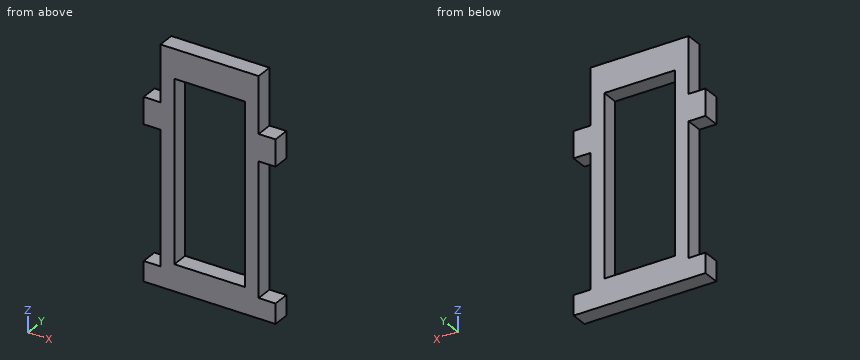
```python
from build123d import *

# Parameters (mm, degrees)
SKETCH1_W           = 53.15
SKETCH1_H           = 135.7
BOSS_EXTRUDE1_DEPTH = 6.35


with BuildPart() as part:
    # Sketch1 → Boss-Extrude1 (new, symmetric)
    with BuildSketch(Plane(origin=(0, 0, 0), x_dir=(1, 0, 0), z_dir=(0, 1, 0))):
        Polygon((-37, -88.675), (-37, -46.325), (-49.7, -46.325), (-49.7, -26.325), (-37, -26.325), (-37, 73.675), (-49.7, 73.675), (-49.7, 88.675), (49.7, 88.675), (49.7, 73.675), (37, 73.675), (37, -26.325), (49.7, -26.325), (49.7, -46.325), (37, -46.325), (37, -88.675), align=None)
        with Locations((0, 1)):
            Rectangle(SKETCH1_W, SKETCH1_H, mode=Mode.SUBTRACT)
    extrude(amount=BOSS_EXTRUDE1_DEPTH, both=True)


solid = part.part
```
Could you check a few things on this model? Use its own coordinates, in mm. Give positions to 0.01 mm unless a question says otherwise; leave off trailing zeros. Loops run counter-clockwise (first coordinate to the right, second up) from the corner with the lowest first, then second, coordinate; pieces in that order, holes last. Notation, with made-up numbers: (7.5, -30) - (28.5, -30) arc R26 cw to (28.5, 1) - close; hole circle Ø9 at (-4.75, 2). An arc over 180 degrees is marked (long way). Use one line per item in the form item = value.
1. I want a section at A-A (y = 2.5). Please give me the cut outline in (x, z) (3 decimals), and give its area (3 significant figures).
Response values:
outline = (-49.7, -88.675) - (49.7, -88.675) - (49.7, -73.675) - (37, -73.675) - (37, 26.325) - (49.7, 26.325) - (49.7, 46.325) - (37, 46.325) - (37, 88.675) - (-37, 88.675) - (-37, 46.325) - (-49.7, 46.325) - (-49.7, 26.325) - (-37, 26.325) - (-37, -73.675) - (-49.7, -73.675) - close; hole (-26.575, -68.85) - (26.575, -68.85) - (26.575, 66.85) - (-26.575, 66.85) - close
area = 6,800 mm²
2. I want a section at C-C (z = 28.5). Please give me the cut outline in (x, y) (3 decimals), and give its area (3 significant figures).
Response values:
outline = (-49.7, -6.35) - (-26.575, -6.35) - (-26.575, 6.35) - (-49.7, 6.35) - close; (26.575, -6.35) - (49.7, -6.35) - (49.7, 6.35) - (26.575, 6.35) - close
area = 587 mm²
3. I want a section at B-B (x = -41). Please give me the cut outline in (y, z) (3 decimals).
Response values:
outline = (-6.35, -88.675) - (6.35, -88.675) - (6.35, -73.675) - (-6.35, -73.675) - close; (-6.35, 26.325) - (6.35, 26.325) - (6.35, 46.325) - (-6.35, 46.325) - close
4. I'm going to push flat-ended pins straight in: pin 1 Ø4 at (y, z) = (1.5, -42.5) entering from +X; pin 2 Ø4 at (y, z) = (-1.5, -26.5) entering from -X; pin 3 Ø4 at (x, y) = (-44.5, 1) entering from +Z (3 decimals); pin 4 Ø5 at (x, z) = (40, 16.5) entering from +Y. Where does each tip first touch, or does it pass through?
Response values:
pin_1 = 37
pin_2 = -37
pin_3 = 46.325
pin_4 = through
5. I need wall thicknesses on probe 1 along Z at (x, y) = (7.5, -3) (3 decimals); probe 2 along X at (y, z) = (4.5, -43.5) (3 decimals); probe 3 along Z at (x, y) = (42, 2) (3 decimals). Which ranges of each line are inside material? Lowest first, please.
Response values:
probe_1 = -88.675 to -68.85, 66.85 to 88.675
probe_2 = -37 to -26.575, 26.575 to 37
probe_3 = -88.675 to -73.675, 26.325 to 46.325
